Here's the drawing with two shaded views (mm, measured from the low corner). I have some questions. A direction names the side the tool comes from. Round coordinates to 2 decimals unless told otherwise and drop trailing zeros. Loops run counter-clockwise (first coordinate to the right, second up) from the corner with the lowest first, then second, coordinate; pieces in that order, holes last. Notation, with made-up numbers: (54, 88.25) -> (86, 88.25) arc R31 cw to (86, 113.25) -> close; hole circle Ø4 at (53, 20.25). An arc over 180 degrees is marked (long way). Use a Markdown table: item, result.
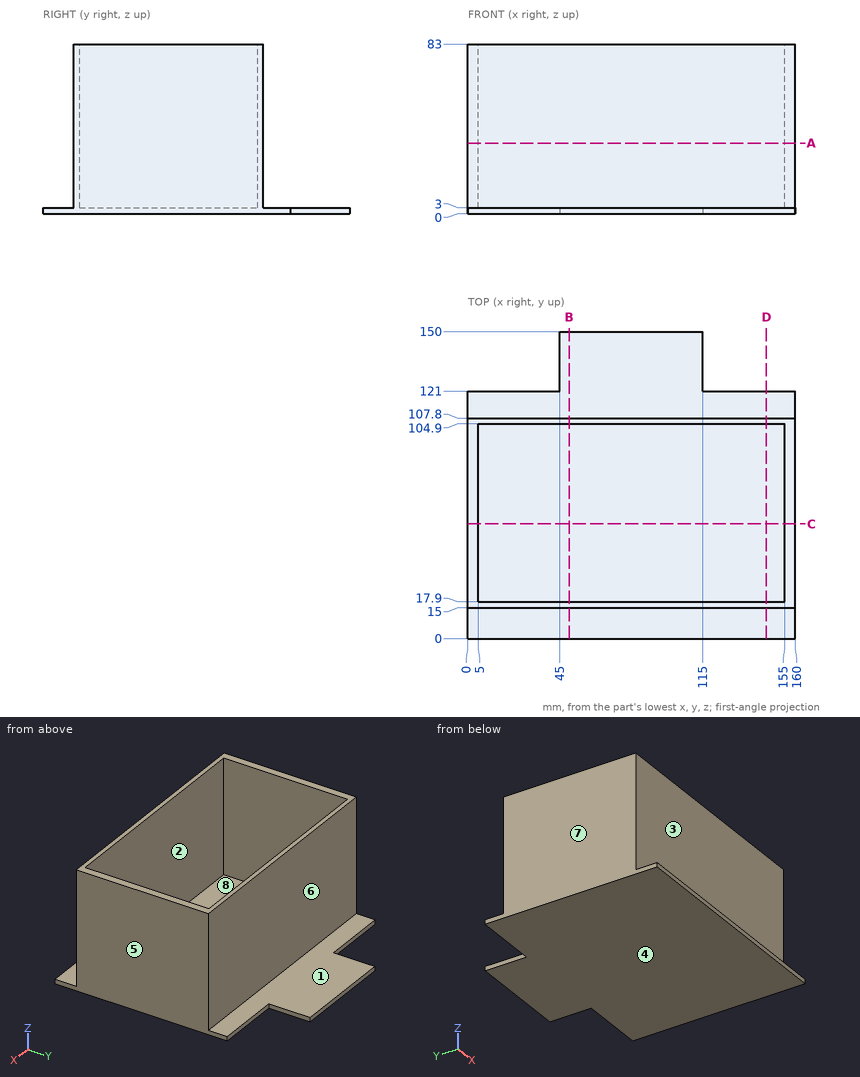
1. If we mould it in two halves opening along X, with no side actions, what happens to the marked faces 5, 6, 7 and 8? For each: +X half, -X half, draft (parallel to the pull), parting line (faces both ways), or undercut.
Answer sheet:
| item | result |
|---|---|
| face 5 | +X half |
| face 6 | draft |
| face 7 | -X half |
| face 8 | undercut |
2. I want a section at D-D (x = 146). Please give me the cut outline in (y, z), plus the area to 3 significant figures.
Answer sheet:
| item | result |
|---|---|
| outline | (0, 0) -> (121, 0) -> (121, 3) -> (107.8, 3) -> (107.8, 83) -> (104.9, 83) -> (104.9, 3) -> (17.9, 3) -> (17.9, 83) -> (15, 83) -> (15, 3) -> (0, 3) -> close |
| area | 827 mm² |
3. I want a section at B-B (x = 49.5). Please give me the cut outline in (y, z).
Answer sheet:
| item | result |
|---|---|
| outline | (0, 0) -> (150, 0) -> (150, 3) -> (107.8, 3) -> (107.8, 83) -> (104.9, 83) -> (104.9, 3) -> (17.9, 3) -> (17.9, 83) -> (15, 83) -> (15, 3) -> (0, 3) -> close |
4. I want a section at C-C (y = 56). Please give me the cut outline in (x, z), plus the area to 3 significant figures.
Answer sheet:
| item | result |
|---|---|
| outline | (0, 0) -> (160, 0) -> (160, 83) -> (155, 83) -> (155, 3) -> (5, 3) -> (5, 83) -> (0, 83) -> close |
| area | 1,280 mm² |
5. I need wall thicknesses on line 1 (X direction, y = 54, z = 67.5); line 2 (Y direction, x = 82, z = 75); line 3 (Z direction, x = 30, y = 57.5). Which ranges of each line are inside material? Lowest first, please.
Answer sheet:
| item | result |
|---|---|
| line 1 | x = 0 to 5, 155 to 160 |
| line 2 | y = 15 to 17.9, 104.9 to 107.8 |
| line 3 | z = 0 to 3 |
6. Which directions (+Z, -Z, +X, -X, +Y, -Y) give clear straight access to the entire face, cutting with the end or side of a thin tool? Please do the marked faces 1, 2, 3 and 4.
Answer sheet:
| item | result |
|---|---|
| face 1 | +Z, +X, -X, +Y |
| face 2 | +Z |
| face 3 | +Z, +X, -X, -Y |
| face 4 | -Z, +X, -X, +Y, -Y |
7. Will these pins go through, and if not, where does the flat tip stop? pin 1 Ø24 at (y, z) = (64, 27.5) entering from -X; pin 2 Ø21 at (x, y) = (105.5, 135) entering from +Z; pin 3 Ø3.5 at (x, z) = (132.5, 1.5) entering from +Y; pin 4 Ø1.5 at (y, z) = (138, 1) entering from -X.
Answer sheet:
| item | result |
|---|---|
| pin 1 | stops at x = 0 |
| pin 2 | stops at z = 3 |
| pin 3 | stops at y = 121 |
| pin 4 | stops at x = 45 |
8. I want a section at A-A (z = 34.5). Please give me the cut outline in (x, y).
Answer sheet:
| item | result |
|---|---|
| outline | (0, 15) -> (160, 15) -> (160, 107.8) -> (0, 107.8) -> close; hole (5, 17.9) -> (155, 17.9) -> (155, 104.9) -> (5, 104.9) -> close |
